For this review, take the finished solid that the model builds, in its own axes (mm). Coordinates: 2 decimals unless noted, no trailing zeros. Write each loop counter-clockwise with the first axis right and the second up, starting at its lowest first coordinate (ties: lowest second). Pieces come first, ordered by that corner, then holes. Notation, with made-up numbers: M 41.5,-38.75 L 73.5,-38.75 A16 cw 73.5,-29.75 Z; hole C 19,67.5 d1. An arc over 180 degrees is marked long. Return JSON: item names as keys, results as strings.
Autodesk Fusion 360 part; units mm, degrees
sketch "long_side" plane through (0, 0, 0) normal (0, 0, 1) x (1, 0, 0)
  line L0 (0, 152.4) -> (285.75, 152.4)
  line L1 (285.75, 152.4) -> (285.75, 0)
  line L2 (285.75, 0) -> (0, 0)
  line L3 (0, 0) -> (0, 152.4)
  circle A0 centre (25.4, 117.4) radius 3.302
  circle A1 centre (25.4, 92) radius 3.302
  circle A2 centre (25.4, 79.3) radius 3.302
  circle A3 centre (25.4, 104.7) radius 3.302
  circle A4 centre (260.35, 117.4) radius 3.302
  circle A5 centre (260.35, 92) radius 3.302
  circle A6 centre (260.35, 104.7) radius 3.302
  circle A7 centre (260.35, 79.3) radius 3.302
  dimension "d1" = 285.75
  dimension "d2" = 152.4
  dimension "d3" = 6.604
  dimension "d55" = 6.604
  dimension "d57" = 6.604
  dimension "d63" = 6.604
  dimension "d75" = 35
  dimension "d76" = 25.4
  dimension "d77" = 12.7
  dimension "d78" = 25.4
  dimension "d79" = 25.4
  dimension "d80" = 25.4
  dimension "d81" = 12.7
  dimension "d82" = 12.7
  dimension "d89" = 6.604
  dimension "d90" = 6.604
  dimension "d91" = 6.604
  dimension "d92" = 6.604
  dimension "d93" = 12.7
  dimension "d94" = 12.7
  dimension "d95" = 12.7
  dimension "d96" = 25.4
  dimension "d97" = 25.4
  dimension "d98" = 25.4
  dimension "d99" = 25.4
  dimension "d100" = 35
extrude "Extrude1" add sketch "long_side" along normal blind 6.35
sketch "Sketch2" plane through (0, 0, 0) normal (0, 0, 1) x (1, 0, 0)
  line L0 (25, 117) -> (25, 104.3) construction
  dimension "d35" = 12.7
1. Wall thickness on L1, parallel to Y at x = 260.35, z = 1.5: over which ranges is the line inside the solid? List them lowest first. Write a range as from..to.
Checks:
{"L1": "0..76, 82.6..88.7, 95.3..101.4, 108..114.1, 120.7..152.4"}
2. Draft analysis for pull direction Y (two halves, no side actions). For faces 1 (the face through (285.75, 77, 3)), 2 (the face through (257.916, 102.468, 3.131)), 3 (the face through (145, 0, 3)), state which applies: +Y half, -Y half, draft (parallel to the pull), parting line (faces both ways), or undercut.
Checks:
{"face 1": "draft", "face 2": "undercut", "face 3": "-Y half"}
3. We need section A-A (y = 92). State the section outline as (x, z) points.
Checks:
{"outline": "M 0,0 L 22.1,0 L 22.1,6.35 L 0,6.35 Z; M 28.7,0 L 257.05,0 L 257.05,6.35 L 28.7,6.35 Z; M 263.65,0 L 285.75,0 L 285.75,6.35 L 263.65,6.35 Z"}
4. We need section B-B (x = 25.4). State the section outline as (y, z) points, plus the area to 3 significant figures.
Checks:
{"outline": "M 0,0 L 76,0 L 76,6.35 L 0,6.35 Z; M 82.6,0 L 88.7,0 L 88.7,6.35 L 82.6,6.35 Z; M 95.3,0 L 101.4,0 L 101.4,6.35 L 95.3,6.35 Z; M 108,0 L 114.1,0 L 114.1,6.35 L 108,6.35 Z; M 120.7,0 L 152.4,0 L 152.4,6.35 L 120.7,6.35 Z", "area": "800 mm2"}
